```python
from build123d import *

# Parameters (mm, degrees)
BOSS_EXTRUDE1_DEPTH = 6
CUT_EXTRUDE1_DEPTH  = 6
SKETCH6_W           = 375
SKETCH6_H           = 15
CUT_EXTRUDE2_DEPTH  = 6
FILLET1_R           = 10
FILLET2_R           = 10
FILLET4_R           = 20
FILLET5_R           = 10
SKETCH7_R           = 12.75
CUT_EXTRUDE3_DEPTH  = 10
SKETCH9_W           = 6
SKETCH9_H           = 40
CUT_EXTRUDE4_DEPTH  = 10


with BuildPart() as part:
    # Sketch3 → Boss-Extrude1 (new body)
    with BuildSketch(Plane(origin=(0, 0, 0), x_dir=(1, 0, 0), z_dir=(0, 1, 0))):
        Polygon((-257.298523245, 138.590313781), (-257.298523245, -71.409686219), (363.88985398, -71.409686219), (363.88985398, 33.590313781), align=None)
    extrude(amount=BOSS_EXTRUDE1_DEPTH)

    # Sketch4 → Cut-Extrude1 (cut)
    with BuildSketch(Plane(origin=(0, 6, 0), x_dir=(1, 0, 0), z_dir=(0, 1, 0))):
        Polygon((-135.235417729, 76.815026044), (-175.235417729, 83.576260082), (-176.251293143, 77.566260082), (-136.251293143, 70.805026044), align=None)
        Polygon((-63.256447035, 64.648359377), (-64.272322449, 58.638359377), (-24.272322449, 51.877125339), (-23.256447035, 57.887125339), align=None)
        Polygon((124.743552965, 32.870559399), (164.743552965, 26.109325362), (163.727677551, 20.099325362), (123.727677551, 26.860559399), align=None)
        Polygon((237.743552965, 13.770073242), (277.743552965, 7.008839205), (276.727677551, 0.998839205), (236.727677551, 7.760073242), align=None)
        Polygon((349.053244456, -15.330412914), (346.517781692, -30.330412914), (352.517781692, -31.34459802), (355.053244456, -16.34459802), align=None)
        Polygon((344.851115025, -40.190545886), (342.315652261, -55.190545886), (348.315652261, -56.204730992), (350.851115025, -41.204730992), align=None)
    extrude(amount=-CUT_EXTRUDE1_DEPTH, mode=Mode.SUBTRACT)

    # Sketch6 → Cut-Extrude2 (cut)
    with BuildSketch(Plane(origin=(0, 6, 0), x_dir=(1, 0, 0), z_dir=(0, 1, 0))):
        with Locations((60.89290198, -63.909686219)):
            Rectangle(SKETCH6_W, SKETCH6_H)
    extrude(amount=-CUT_EXTRUDE2_DEPTH, mode=Mode.SUBTRACT)

    # Fillet1
    fillet1_edges = [part.edges().sort_by_distance(p)[0] for p in [
        (-126.60709802, 3, 56.409686219),
    ]]
    fillet(fillet1_edges, radius=FILLET1_R)

    # Fillet2
    fillet2_edges = [part.edges().sort_by_distance(p)[0] for p in [
        (248.39290198, 3, 56.409686219),
    ]]
    fillet(fillet2_edges, radius=FILLET2_R)

    # Fillet4
    fillet4_edges = [part.edges().sort_by_distance(p)[0] for p in [
        (363.88985398, 3, -33.590313781),
        (363.88985398, 3, 71.409686219),
        (-257.298523245, 3, 71.409686219),
        (-257.298523245, 3, -138.590313781),
    ]]
    fillet(fillet4_edges, radius=FILLET4_R)

    # Fillet5
    fillet5_edges = [part.edges().sort_by_distance(p)[0] for p in [
        (248.39290198, 3, 71.409686219),
        (-126.60709802, 3, 71.409686219),
    ]]
    fillet(fillet5_edges, radius=FILLET5_R)

    # Sketch7 → Cut-Extrude3 (cut)
    with BuildSketch(Plane(origin=(0, 6, 0), x_dir=(1, 0, 0), z_dir=(0, 1, 0))):
        with Locations(Location((193.372247473, -6.409686219, 0), (0, 0, 270))):
            Circle(SKETCH7_R)
    extrude(amount=-CUT_EXTRUDE3_DEPTH, mode=Mode.SUBTRACT)

    # Sketch9 → Cut-Extrude4 (cut)
    with BuildSketch(Plane(origin=(0, 6, 0), x_dir=(1, 0, 0), z_dir=(0, 1, 0))):
        with Locations((-254.298523245, 48.590313781)):
            Rectangle(SKETCH9_W, SKETCH9_H)
        with Locations((-254.298523245, -11.409686219)):
            Rectangle(SKETCH9_W, SKETCH9_H)
    extrude(amount=-CUT_EXTRUDE4_DEPTH, mode=Mode.SUBTRACT)


solid = part.part
```
Could you check a few things on this model? Use its own coordinates, in mm. Give positions to 0.01 mm unless a question says otherwise; leave off trailing zeros. Order: outer loops, then holes, each group sorted by start corner. A loop starts at its lowest first (then second) coordinate and runs counter-clockwise, first axis right, second up.
Q1. I'm going to push flat-ended pins straight in: P1, Ø3, axis at x = -254.5, y = 2.5, coming from the -Z side; P2, Ø3, axis at y = 2.5, z = -55, coming from the -X side; P3, Ø1.8, axis at x = -254.5, y = 4.5, coming from the +Z side. Where does each tip first touch, or does it pass through?
Q2. We'd pull the mould along Z, two halves only. Please class faces 1 (the flat face through (-20, 0, -10)), 2 (the flat face through (60.7, 2.96, -84.84)), 3 (the cylindrical face through (180.925, 3.042, 3.646)), 4 (the cylindrical face through (357.876, 3.042, 65.706)): +Z half, -Z half, draft (parallel to the pull), parting line (faces both ways), or undercut.
Q3. If I drill on line 1 along Z through (x, y) = (-35, 1) (3 decimals); line 2 along X through (y, z) = (0.75, 13); line 3 along Z through (x, y) = (187.5, 5), over which ranges is the centre line in solid material (lowest first)?
Q4. Suppose I cut it at C-C, the plane x = 270.5. Write out the boundary of the cut face in (y, z).
Q5. Suppose I cut it at D-D, the plane z = -91. Write out the boundary of the cut face in (x, y), and give its area (3 significant figures).
Q6. Suppose I cut it at A-A, the plane x = -40. Write out the boundary of the cut face in (y, z).
Q7. Suppose I cut it at B-B, the plane y = 4.5. Count the separate pieces of the cut face and the enclosed holes in it, and give its area (3 significant figures).
Solution:
1. P1: stops at z = -127.31
1. P2: stops at x = -251.3
1. P3: stops at z = 63
2. face 1: draft
2. face 2: -Z half
2. face 3: undercut
2. face 4: +Z half
3. line 1: z = -101.015 to -59.872, -53.69 to 56.41
3. line 2: x = -251.3 to 182.46, 204.29 to 363.89
3. line 3: z = -63.41 to -4.91, 17.73 to 56.41
4. outline: (0, -49.38) - (6, -49.38) - (6, -8.23) - (0, -8.23) - close; (0, -2.05) - (6, -2.05) - (6, 71.41) - (0, 71.41) - close
5. outline: (-257.3, 0) - (24.25, 0) - (24.25, 6) - (-257.3, 6) - close
5. area: 1,690 mm2
6. outline: (0, -101.86) - (6, -101.86) - (6, -60.72) - (0, -60.72) - close; (0, -54.54) - (6, -54.54) - (6, 56.41) - (0, 56.41) - close
7. separate pieces: 1
7. enclosed holes: 7
7. area: 89,700 mm2
